Autodesk Inventor part; units mm, degrees
ref_plane "YZ Plane" through (0, 0, 0) normal (1, 0, 0) x (0, 1, 0)
ref_plane "XZ Plane" through (0, 0, 0) normal (0, 1, 0) x (-1, 0, 0)
ref_plane "XY Plane" through (0, 0, 0) normal (0, 0, 1) x (1, 0, 0)
sketch "Esquisse1" plane through (0, 0, 0) normal (0, 1, 0) x (-1, 0, 0)
  line L0 (0, 0) -> (150, 0)
  line L1 (150, 0) -> (150, -40)
  line L2 (150, -40) -> (0, -40)
  line L3 (0, -40) -> (0, 0)
  line L4 (150, -20) -> (0, -20) construction
  line L5 (150, -10) -> (0, -10) construction
  line L6 (150, -30) -> (0, -30) construction
  circle A0 centre (95, -5) radius 2.5
  line L7 (75, 0) -> (75, -40) construction
  circle A1 centre (55, -5) radius 2.5
  circle A2 centre (95, -35) radius 2.5
  circle A3 centre (55, -35) radius 2.5
  circle A4 centre (140, -5) radius 2.5
  circle A5 centre (140, -35) radius 2.5
  circle A6 centre (10, -5) radius 2.5
  circle A7 centre (10, -35) radius 2.5
  dimension "d0" = 150
  dimension "d2" = 10
  dimension "d3" = 10
  dimension "d4" = 5
  dimension "d12" = 5
  dimension "d13" = 20
  dimension "d14" = 20
  dimension "d15" = 5
  dimension "d16" = 10
  dimension "d17" = 5
extrude "Extrusion1" add sketch "Esquisse1" along normal blind 6
equation "\"d3\" = d2"
equation "\"d17\" = d12"
properties part number "hold_motor_bottom" material "Bois (cerisier)"
The listing builds one solid part. Answer for the finished solid, in the listing's coordinates (mm). Coordinates: 2 decimals unless noted, no trailing zeros. Loops run counter-clockwise (first coordinate to the right, second up) from the corner with the lowest first, then second, coordinate; pieces in that order, holes last. Notation, with made-up numbers: (73.25, -11.5) -> (126.25, -11.5) arc R19 cw to (126.25, 1.5) -> close; hole circle Ø2 at (51, 52). An arc over 180 degrees is marked (long way). Answer in a Markdown table with one row per item. Add a question column.
1. Flat-ended cylindrical pins translate along their axes: P1, Ø4, axis at x = -10, z = -35, coming from the -Y side; P2, Ø6, axis at x = -95, z = -5, coming from the -Y side. Find the tip coordinate at first contact, or state that the pin passes through.
2. The part is cut by section A-A, the plane y = 1.25. Count the separate pieces of the cut face and the enclosed holes in it, then the cut area to 3 significant figures.
3. Consider line 1 (Z direction, x = -95, y = 3.3); line 2 (X direction, y = 1, z = -6); line 3 (X direction, y = 4.65, z = -36.5). Determine where each line is inside the solid, lowest interval first. Write a range as [from, to].
4. The part is cut by section C-C, the plane x = -10. Write down the section's boundary in (y, z).
5. The part is cut by section B-B, the plane z = -35. Write down the section's boundary in (x, y), then the cut area to 3 significant figures.
6. Determine the mould class of faces 1 (the flat face through (0, 3, -20)), 2 (the cylindrical face through (-142.385, 2.958, -35.751)), 3 (the cylindrical face through (-57.31, 2.96, -34.04)), 4 (the flat face through (-74, 6, -20)) for opening direction X: +X half, -X half, draft (parallel to the pull), parting line (faces both ways), or undercut.
Answer below:
| question | item | result |
|---|---|---|
| 1 | P1 | through |
| 1 | P2 | y = 0 |
| 2 | separate pieces | 1 |
| 2 | enclosed holes | 8 |
| 2 | area | 5,840 mm2 |
| 3 | line 1 | [-40, -37.5], [-32.5, -7.5], [-2.5, 0] |
| 3 | line 2 | [-150, -142.29], [-137.71, -97.29], [-92.71, -57.29], [-52.71, -12.29], [-7.71, 0] |
| 3 | line 3 | [-150, -142], [-138, -97], [-93, -57], [-53, -12], [-8, 0] |
| 4 | outline | (0, -40) -> (6, -40) -> (6, -37.5) -> (0, -37.5) -> close; (0, -32.5) -> (6, -32.5) -> (6, -7.5) -> (0, -7.5) -> close; (0, -2.5) -> (6, -2.5) -> (6, 0) -> (0, 0) -> close |
| 5 | outline | (-150, 0) -> (-142.5, 0) -> (-142.5, 6) -> (-150, 6) -> close; (-137.5, 0) -> (-97.5, 0) -> (-97.5, 6) -> (-137.5, 6) -> close; (-92.5, 0) -> (-57.5, 0) -> (-57.5, 6) -> (-92.5, 6) -> close; (-52.5, 0) -> (-12.5, 0) -> (-12.5, 6) -> (-52.5, 6) -> close; (-7.5, 0) -> (0, 0) -> (0, 6) -> (-7.5, 6) -> close |
| 5 | area | 780 mm2 |
| 6 | face 1 | +X half |
| 6 | face 2 | undercut |
| 6 | face 3 | undercut |
| 6 | face 4 | draft |
